For this review, take the finished solid that the model builds, in its own axes (mm). Round coordinates to 2 decimals unless told otherwise and drop trailing zeros. Order: outer loops, then holes, each group sorted by start corner. A loop starts at its lowest first (then second) coordinate and runs counter-clockwise, first axis right, second up. Notation, with made-up numbers: M -30.5,-2.75 L -4.5,-2.75 A18 cw -4.5,7.25 Z; hole C 71,61 d1. An arc over 180 degrees is marked long. Use a Markdown table: item, result.
Autodesk Inventor part; units mm, degrees
ref_plane "YZ Plane" through (0, 0, 0) normal (1, 0, 0) x (0, 1, 0)
ref_plane "XZ Plane" through (0, 0, 0) normal (0, 1, 0) x (-1, 0, 0)
ref_plane "XY Plane" through (0, 0, 0) normal (0, 0, 1) x (1, 0, 0)
sketch "Sketch1" plane through (0, 0, 0) normal (0, 1, 0) x (-1, 0, 0)
  circle A0 centre (0, 0) radius 40
  circle A1 centre (0, 0) radius 35
  line L0 (2.3, 32.9859) -> (2.3, 40)
  line L1 (21.9637, 27.3435) -> (25.5064, 30.8949)
  line L2 (21.9637, 27.3435) -> (21.9123, 27.292)
  line L3 (26.5671, 29.8368) -> (23.0244, 26.2855)
  line L4 (26.5671, 29.8368) -> (26.6021, 29.8719)
  line L5 (25.4356, 30.9655) -> (21.8929, 27.4142)
  line L6 (21.8929, 27.4142) -> (21.8415, 27.3626)
  line L7 (21.8415, 27.3626) -> (21.8337, 27.3548)
  line L8 (23.0952, 26.2148) -> (26.6379, 29.7662)
  line L9 (26.6379, 29.7662) -> (26.6729, 29.8013)
  line L10 (26.6729, 29.8013) -> (26.6768, 29.8052)
  circle A2 centre (0, 0) radius 42
  line L11 (2.4, 32.9859) -> (2.4, 39.9955)
  line L12 (34.7391, 5.0137) -> (39.7719, 5.0137)
  line L13 (39.7719, 3.5174) -> (34.7391, 3.5174)
  line L14 (34.7391, 5.1137) -> (39.7645, 5.1137)
  line L15 (39.7719, 3.4174) -> (34.7391, 3.4174)
  line L16 (34.7391, 5.1137) -> (34.6244, 5.1137)
  line L17 (39.7719, 3.4174) -> (39.8538, 3.4174)
  line L18 (23, -32.7261) -> (23, -26.3818)
  line L19 (23.1, -32.7236) -> (23.1, -26.3856)
  line L20 (23.1, -26.3856) -> (23.1, -26.2943)
  line L21 (21.5, -32.7261) -> (21.5, -26.3818)
  line L22 (21.4, -32.723) -> (21.4, -26.3818)
  line L23 (21.4, -32.723) -> (21.4, -33.7941)
  line L24 (0.75, -35) -> (0.75, -40)
  line L25 (0.85, -35.0011) -> (0.85, -39.8733)
  line L26 (0.85, -35.0011) -> (0.85, -34.9897)
  line L27 (0.85, -39.8733) -> (0.85, -41.9914)
  line L28 (2.4, 39.9955) -> (2.4, 41.9314)
  line L29 (23, -32.7261) -> (21.5, -32.7261)
  line L30 (22.8571, -32.8261) -> (21.4, -32.8261)
  line L31 (23.1, -32.7236) -> (23.1, -32.8261)
  line L32 (22.8571, -32.8261) -> (23.1, -32.8261)
  line L33 (39.7719, 5.0137) -> (39.7719, 3.5174)
  line L34 (39.8719, 3.4174) -> (39.8719, 5.1137)
  line L35 (39.7645, 5.1137) -> (39.8719, 5.1137)
  line L36 (39.8719, 3.4174) -> (39.8538, 3.4174)
  point P0 (2.4, 34.9176)
  point P1 (25.3839, 30.9137)
  point P2 (23.1396, 26.2594)
  point P3 (39.6718, 5.1137)
  point P4 (34.8328, 3.4174)
  point P5 (23.1, -32.6556)
  point P6 (21.4, -27.6955)
  dimension "d0" = 0.1
  dimension "d1" = 0.1
  dimension "d2" = 2
  dimension "d3" = 0.1
  dimension "d4" = 0.1
  dimension "d5" = 0.1
  dimension "d6" = 0.1
  dimension "d7" = 0.1
  dimension "d8" = 0.1
  dimension "d13" = 0.1
  dimension "d16" = 0.1
extrude "Extrusion1" add sketch "Sketch1" along normal blind 3 contours A0 L19 L20 A1 L15 L17 | A0 L36 L34 L35 L14 L11 L28 A2 L27 L32 L31 L19 | L14 L16 A1 L8 L9 L10 A0 | A0 L27 L25 L26 A1 L22 L23 | L5 L6 L7 A1 L11 A0
sketch "Sketch2" plane through (0, 3, 0) normal (0, 1, 0) x (1, 0, 0)
  line L0 (-21.4, 33.7941) -> (-21.4, 27.6955)
  arc A0 (-0.85, 34.9897) -> (-21.4, 27.6955) centre (0, 0) ccw
  line L1 (-25.3839, -30.9137) -> (-16.4117, -30.9137)
  arc A1 (-21.8337, -27.3548) -> (-2.4, -34.9176) centre (0, 0) ccw
  line L2 (-21.8337, -27.3548) -> (-25.3839, -30.9137)
  line L3 (-23.1, 32.8261) -> (-12.1427, 32.8261)
  point P0 (-9.1082, 33.7941)
  point P1 (-21.4, 32.8261)
extrude "Extrusion2" cut sketch "Sketch2" against normal through all
sketch "Sketch3" plane through (0, 3, 0) normal (0, 1, 0) x (1, 0, 0)
  line L0 (-21.4, 33.7941) -> (-21.4, 32.8261)
  line L1 (-22.8571, 32.8261) -> (-21.4, 32.8261)
  arc A0 (-21.4, 33.7941) -> (-22.8571, 32.8261) centre (0, 0) ccw
extrude "Extrusion3" add sketch "Sketch3" against normal blind 3
equation "\"d0\" = slack"
equation "\"d1\" = slack"
equation "\"d3\" = slack"
equation "\"d4\" = slack"
equation "\"d5\" = slack"
equation "\"d6\" = slack"
equation "\"d7\" = slack"
equation "\"d8\" = slack"
equation "\"d13\" = slack"
equation "\"d16\" = slack"
equation "\"d9\" = thicc"
equation "\"d14\" = thicc"
equation "\"slack\" = 0.1"
equation "\"thicc\" = 3"
properties part number "Front_aligner"
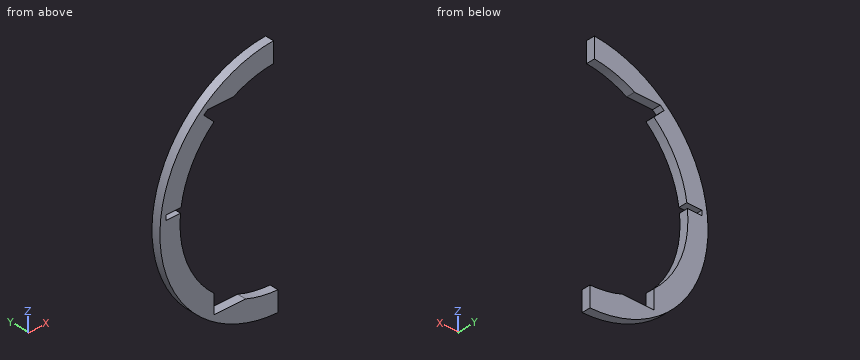
Q1. Add section D-D (z = 0). Write out the cut boundary in (x, y).
Determined:
| item | result |
|---|---|
| outline | M -42,0 L -35,0 L -35,3 L -42,3 Z |
Q2. Add section B-B (x = -37). Write out the cut boundary in (y, z).
Determined:
| item | result |
|---|---|
| outline | M 0,-19.87 L 3,-19.87 L 3,3.42 L 0,3.42 Z; M 0,5.11 L 3,5.11 L 3,19.87 L 0,19.87 Z |
Q3. Wall thickness on line 1 along Z through (x, y) = (-26.5, 1.65); line 2 along Z through (x, y) = (-5, 1.6); line 3 along Z through (x, y) = (-18, 2.05): over which ranges is each line inside the solid? List them lowest first. Write a range as [from, to].
Determined:
| item | result |
|---|---|
| line 1 | z = [-32.58, -22.86], [22.86, 29.63], [29.96, 32.58] |
| line 2 | z = [-41.7, -34.64], [34.64, 41.7] |
| line 3 | z = [-37.95, -32.83], [30.91, 37.95] |
Q4. Add section A-A (x = -24.5). Write out the cut boundary in (y, z) (3 decimals).
Determined:
| item | result |
|---|---|
| outline | M 0,-34.114 L 3,-34.114 L 3,-24.995 L 0,-24.995 Z; M 0,24.995 L 3,24.995 L 3,27.623 L 0,27.623 Z; M 0,30.914 L 3,30.914 L 3,34.114 L 0,34.114 Z |
Q5. Clearance check with flat-ended pins moving along their axes: pin 1 (1.5 mm diameter, centred on y = 0.5, z = -9.5, fed in from -X); pin 2 (12 mm diameter, centred on x = -32.5, z = 11.5, fed in from -Y); pin 3 (1.5 mm diameter, centred on x = -37, y = 1.5, fed in from -Z); pin 4 (1 mm diameter, centred on x = -11, y = 2.5, fed in from +Z). State where each tip first meets the part, or that it passes through.
Determined:
| item | result |
|---|---|
| pin 1 | stops at x = -41.08 |
| pin 2 | stops at y = 0 |
| pin 3 | stops at z = -21.21 |
| pin 4 | stops at z = 40.67 |
